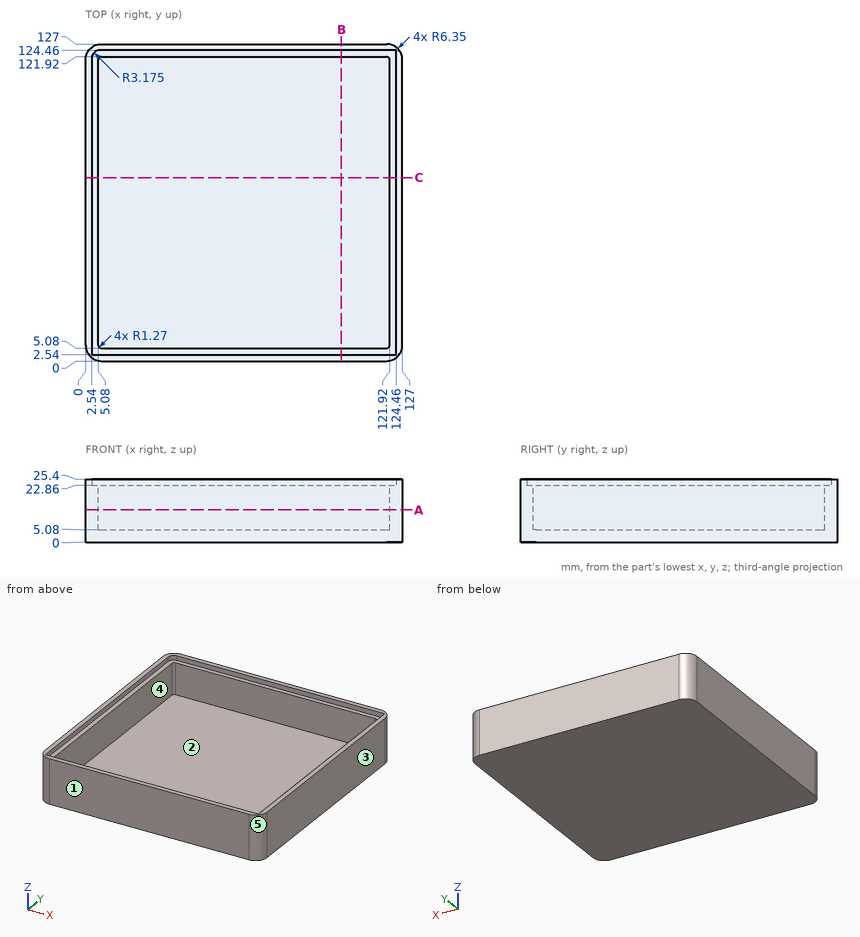
Could you check a few things on this drawing? It's one solid part, dimensions in mm from its lowest x, y, z. A direction names the side the tool comes from. Coordinates: 2 decimals unless noted, no trailing zeros. Order: outer loops, then holes, each group sorted by start corner. A loop starts at its lowest first (then second) coordinate and runs counter-clockwise, first axis right, second up. Notation, with made-up numbers: (81.25, 58) -> (117.25, 58) arc R20 cw to (117.25, 68) -> close; hole circle Ø5 at (-0.75, -16). An arc over 180 degrees is marked (long way). Answer in a Markdown table with one row per item.
(1) I want a section at B-B on x = 102.5. List the corners of the cut face in (y, z) for me, then the cut area to 3 significant figures.
Answer key:
| item | result |
|---|---|
| outline | (0, 0) -> (127, 0) -> (127, 25.4) -> (124.46, 25.4) -> (124.46, 22.86) -> (121.92, 22.86) -> (121.92, 5.08) -> (5.08, 5.08) -> (5.08, 22.86) -> (2.54, 22.86) -> (2.54, 25.4) -> (0, 25.4) -> close |
| area | 839 mm^2 |
(2) I want a section at A-A on z = 13. List the corners of the cut face in (x, y) for me.
Answer key:
| item | result |
|---|---|
| outline | (0, 6.35) arc R6.35 ccw to (6.35, 0) -> (120.65, 0) arc R6.35 ccw to (127, 6.35) -> (127, 120.65) arc R6.35 ccw to (120.65, 127) -> (6.35, 127) arc R6.35 ccw to (0, 120.65) -> close; hole (5.08, 6.35) arc R1.27 ccw to (6.35, 5.08) -> (120.65, 5.08) arc R1.27 ccw to (121.92, 6.35) -> (121.92, 120.65) arc R1.27 ccw to (120.65, 121.92) -> (6.35, 121.92) arc R1.27 ccw to (5.08, 120.65) -> close |
(3) Please list where these lines run through material, in increasing order: probe 1 along Y at (x, z) = (41.5, 19.5); probe 2 along X at (y, z) = (88.5, 24.75).
Answer key:
| item | result |
|---|---|
| probe 1 | 0 to 5.08, 121.92 to 127 |
| probe 2 | 0 to 2.54, 124.46 to 127 |
(4) Thinking about a two-plate mould opening in Y: for the marked faces 3, 4 and 5, which applies, +Y half, -Y half, draft (parallel to the pull), parting line (faces both ways), or undercut?
Answer key:
| item | result |
|---|---|
| face 3 | draft |
| face 4 | undercut |
| face 5 | -Y half |
(5) Will this pin go through, and if not, where does the flat tip stop? pin 1 Ø6 at (x, y) = (27, 81) entering from +Z.
Answer key:
| item | result |
|---|---|
| pin 1 | z = 5.08 |
(6) On a 3-axis mill with a long thin cutter (end or side, diameter ignored), from which of +Z, -Z, +X, -X, +Y, -Y can I reach the whole of each face in a straight line? I mean the marked faces 1 and 2. Say none if no direction works.
Answer key:
| item | result |
|---|---|
| face 1 | +Z, -Z, +X, -X, -Y |
| face 2 | +Z |
